```python
from build123d import *

# Parameters (mm, degrees)
CHAMFER1_SIZE = 0.762
CHAMFER2_SIZE = 0.762


with BuildPart() as part:
    # Sketch3 → Revolve1 (revolve)
    with BuildSketch(Plane.XY, mode=Mode.PRIVATE) as revolve1_sk:
        Polygon((-32.131, 0), (32.131, 0), (32.131, 2.413), (19.431, 2.413), (19.431, 3.175), (-19.431, 3.175), (-19.431, 2.413), (-32.131, 2.413), align=None)
    revolve(revolve1_sk.sketch.rotate(Axis((-32.131, 0, 0), (1, 0, 0)), 90), axis=Axis((-32.131, 0, 0), (1, 0, 0)))

    # Chamfer1
    chamfer1_edges = [part.edges().sort_by_distance(p)[0] for p in [
        (-32.131, 0, -2.413),
    ]]
    chamfer(chamfer1_edges, length=CHAMFER1_SIZE)

    # Chamfer2
    chamfer2_edges = [part.edges().sort_by_distance(p)[0] for p in [
        (32.131, 0, -2.413),
    ]]
    chamfer(chamfer2_edges, length=CHAMFER2_SIZE)


solid = part.part
```
Part model, mm, in its own coordinate system. A direction names the side the tool comes from. Coordinates: 2 decimals unless noted, no trailing zeros. Loops run counter-clockwise (first coordinate to the right, second up) from the corner with the lowest first, then second, coordinate; pieces in that order, holes last. Notation, with made-up numbers: (-20.5, -39) - (-5.5, -39) arc R23 cw to (-5.5, -26) - close; hole circle Ø5 at (9, 64). An arc over 180 degrees is marked (long way). Write item = value, one per line. Start each with the question number.
Item 1: Flat gauge pins, fed straight in: pin 1 Ø3 at (x, z) = (21, -1.5) entering from -Y; pin 2 Ø3 at (y, z) = (-2.5, 2) entering from +X. Where does each tip first touch, or does it go through?
Item 2: Cut at D-D, the plane x = -15.5. Give the cut face in (y, z) (3 decimals).
Item 3: Cut at C-C, the plane x = 20. Give the cut face in (y, z).
Item 4: 3-axis set-ups, long thin cutter, end or side, ignore diameter. For faces 1 (the flat face through (32.131, 0, 0)), 2 (the cylindrical face through (-25.484, 1.468, -1.915)), 3 (the cylindrical face through (25.316, 1.468, -1.915)): which of +Z, -Z, +X, -X, +Y, -Y reach the whole face in a straight line?
Item 5: Cut at A-A, the plane y = 0. Give the cut face in (x, z) (3 decimals).
Item 6: Wall check: L1, parallel to X at y = 2.75, z = 0.5; L2, parallel to Y at x = 18.5, z = -1. Give the ranges that are in metal, low to high. Write a range as from..to.
The answers:
q1.pin_1 = -2.41
q1.pin_2 = 32.08
q2.outline = circle Ø6.35 at (0, 0)
q3.outline = circle Ø4.83 at (0, 0)
q4.face_1 = +Z, -Z, +X, +Y, -Y
q4.face_2 = -X
q4.face_3 = +X
q5.outline = (-32.131, -1.651) - (-31.369, -2.413) - (-19.431, -2.413) - (-19.431, -3.175) - (19.431, -3.175) - (19.431, -2.413) - (31.369, -2.413) - (32.131, -1.651) - (32.131, 1.651) - (31.369, 2.413) - (19.431, 2.413) - (19.431, 3.175) - (-19.431, 3.175) - (-19.431, 2.413) - (-31.369, 2.413) - (-32.131, 1.651) - close
q6.L1 = -19.43..19.43
q6.L2 = -3.01..3.01
